from build123d import *

# Parameters (mm, degrees)
F1_DEPTH = 6.9342
F2_SCALE = 0.5
F3_R     = 11.0998
F4_DEPTH = 25.4


with BuildPart() as f1:
    # F0 (on Top) → F1 (new body)
    with BuildSketch(Plane.XY):
        Polygon((-75.6856215453, 61.495130631), (-103.0089063366, 52.4619456377), (-80.056669942, 23.3529183213), (-71.3269899235, 27.5684058967), (-77.7287712085, 20.0368960855), (-54.0167096295, -6.7615591093), (-43.9553417197, -1.0685261115), (-51.4435459742, -10.473888544), (-33.5140929693, -30.3097563356), (-21.7221314678, -19.7887847189), (-25.1305638593, -42.9484921738), (0, -68.3683384545), (25.6179132403, -43.0419616731), (22.0779453622, -19.4793259238), (33.8894912196, -30.2508644393), (51.9251031665, -10.473888544), (44.763548994, -0.9251482466), (54.5851095356, -6.9272132295), (78.2306868312, 20.0916471891), (72.0478651347, 27.7012792084), (80.7445831733, 23.3529183213), (103.7288850297, 52.37963034), (76.0650205074, 61.495130631), (20.2681753259, 17.5302260523), (7.5507578667, 37.5718755511), (-15.3496812645, 37.5718755511), (-22.6703244303, 30.3177857753), (-6.6980118564, 29.7188239429), (-20.0065281242, 17.5278745592), align=None)
    extrude(amount=F1_DEPTH)


with BuildPart() as f1_1:
    # F2: moved
    add(f1.part.scale(F2_SCALE))

    # F3 (on face) → F4 (cut)
    with BuildSketch(Plane.XY.offset(3.4671)):
        with Locations((0, -1.8054934917)):
            Circle(F3_R)
    extrude(amount=-F4_DEPTH, mode=Mode.SUBTRACT)


solid = f1_1.part
Work out the finished part from the listing and answer in its coordinate system (mm). A direction names the side the tool comes from. Coordinates: 2 decimals unless noted, no trailing zeros. Write each loop counter-clockwise with the first axis right and the second up, starting at its lowest first coordinate (ties: lowest second). Pieces come first, ordered by that corner, then holes. Notation, with made-up numbers: M 28,5.5 L 78,5.5 A4 cw 78,11.5 Z; hole C 27,10.5 d4. An arc over 180 degrees is marked long. Write item = value, one per line.
1. Flat-ended cylindrical pins translate along their axes: pin 1 (1 mm diameter, centred on y = 13, z = 0.5, fed in from -X); pin 2 (2 mm diameter, centred on x = -26.5, z = 2.5, fed in from +Y); pin 3 (1.7 mm diameter, centred on x = -1, z = 1, fed in from +Y). Find the tip coordinate at first contact, or state that the pin passes through.
Solution:
pin_1 = -41.47
pin_2 = 22.58
pin_3 = 18.79
2. The part is cut by section D-D (x = -19). Determine the outline of the cut face in (y, z).
Solution:
outline = M -12.67,0 L 15.87,0 L 15.87,3.47 L -12.67,3.47 Z
3. The part is cut by section B-B (y = 25). Determine the outline of the cut face in (x, z).
Solution:
outline = M -50.53,0 L -30.56,0 L -30.56,3.47 L -50.53,3.47 Z; M 30.74,0 L 50.92,0 L 50.92,3.47 L 30.74,3.47 Z
4. Determine the mould class of faces 1 (the face through (-2, 18.786, 2)), 2 (the face through (0, 10, 0)), 3 (the face through (21.39, -10.25, 1.71)) for opening direction X: released by +X, released by -X, zero draft, split by the parting line, or undercut.
Solution:
face_1 = undercut
face_2 = zero draft
face_3 = released by +X
5. Straight lines are drawn through the part: line 1 (Y direction, x = 0, z = 2.75); line 2 (X direction, y = -15, z = 0.7); line 3 (X direction, y = -12, z = 0.2). For each, find the intervals that lie inside material, in ascending order. Write a range as from..to.
Solution:
line_1 = -34.18..-12.91, 9.29..18.79
line_2 = -16.9..-16.58, -11.61..11.83, 16.81..17.06
line_3 = -19.61..-13.22, -11.17..-4.39, 4.39..11.38, 13.52..19.79
6. The part is cut by section A-A (x = -1.5). Determine the outline of the cut face in (y, z).
Solution:
outline = M -32.67,0 L -12.8,0 L -12.8,3.47 L -32.67,3.47 Z; M 9.19,0 L 18.79,0 L 18.79,3.47 L 9.19,3.47 Z
7. For faces 4 (the face through (-6.63, 11.854, 1.709)), 5 (the face through (33.121, 3.197, 1.709)), 6 (the face through (24.28, 19.91, 1.71)), determine the directions among +Z, -Z, +X, -X, +Y, -Y from which every point of the face is accessible in a straight line to the end or side of a thin tool.
Solution:
face_4 = +Z, -Z
face_5 = +Z, -Z, +X, -Y
face_6 = +Z, -Z, +Y
